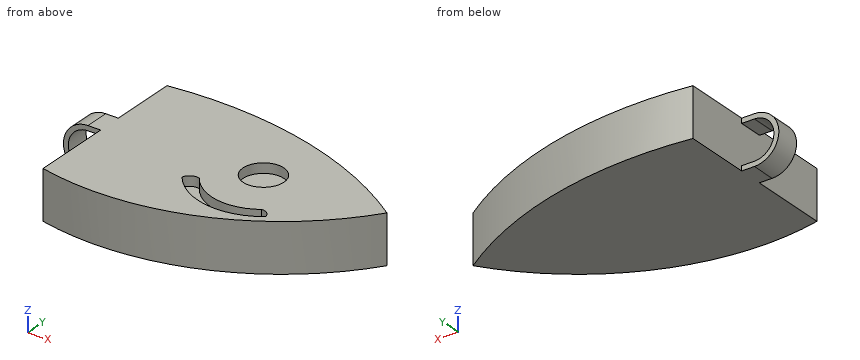
```python
from build123d import *

# Parameters (mm, degrees)
EXTRUDE_1_DEPTH     = 10
SKETCH_2_R          = 4.182683646
CUT_EXTRUDE_1_DEPTH = 2
CUT_EXTRUDE_2_DEPTH = 2
EXTRUDE_2_DEPTH     = 5
CUT_EXTRUDE_4_DEPTH = 5


with BuildPart() as part:
    # 草圖1 → 填料-伸長1 (new body)
    with BuildSketch(Plane.XY):
        with BuildLine():
            Line((-54.969523774, 13.719179235), (-54.969523774, -21.22476033))
            ThreePointArc((-54.969523774, -21.22476033), (-24.214711694, -19.081408744), (0, 0))
            ThreePointArc((0, 0), (-26.203666434, 11.992637721), (-54.969523774, 13.719179235))
        make_face()
    extrude(amount=EXTRUDE_1_DEPTH)

    # 草圖2 → 除料-伸長1 (cut)
    with BuildSketch(Plane(origin=(-3.59892411, 0, 10), x_dir=(1, 0, 0), z_dir=(0, 0, 1))):
        with Locations((-20.534055943, -1.585781503)):
            Circle(SKETCH_2_R)
    extrude(amount=-CUT_EXTRUDE_1_DEPTH, mode=Mode.SUBTRACT)

    # 草圖3 → 除料-伸長2 (cut)
    with BuildSketch(Plane(origin=(-4.498655138, 1.869163063, 10), x_dir=(1, 0, 0), z_dir=(0, 0, 1))):
        with BuildLine():
            ThreePointArc((-30.154301824, -11.927771695), (-21.15958892, -17.29086396), (-11.007087523, -14.722920379))
            ThreePointArc((-11.007087523, -14.722920379), (-11.654774806, -13.513501992), (-12.967946819, -13.116298119))
            ThreePointArc((-12.967946819, -13.116298119), (-20.827814666, -14.857391145), (-27.616719206, -10.530763976))
            ThreePointArc((-27.616719206, -10.530763976), (-29.174840287, -10.703717268), (-30.154301824, -11.927771695))
        make_face()
    extrude(amount=-CUT_EXTRUDE_2_DEPTH, mode=Mode.SUBTRACT)

    # 草圖4 → 填料-伸長2 (add)
    with BuildSketch(Plane(origin=(0, 0, 0), x_dir=(1, 0, 0), z_dir=(0, 1, 0))):
        with BuildLine():
            Line((-54.969523774, 0), (-57.578183819, 0))
            ThreePointArc((-57.578183819, 0), (-62.578183819, -5), (-57.578183819, -10))
            Line((-57.578183819, -10), (-54.969523774, -10))
            Line((-54.969523774, -10), (-54.969523774, 0))
        make_face()
    extrude(amount=-EXTRUDE_2_DEPTH)

    # 草圖5 → 除料-伸長4 (cut)
    with BuildSketch(Plane(origin=(0, 0, 0), x_dir=(1, 0, 0), z_dir=(0, 1, 0))):
        with BuildLine():
            Line((-54.969523774, -1), (-57.578183819, -1))
            ThreePointArc((-57.578183819, -1), (-61.578183819, -5), (-57.578183819, -9))
            Line((-57.578183819, -9), (-54.969523774, -9))
            Line((-54.969523774, -9), (-54.969523774, -1))
        make_face()
    extrude(amount=-CUT_EXTRUDE_4_DEPTH, mode=Mode.SUBTRACT)


solid = part.part
```
Model file for the job. Use its own axes, mm. Coordinates: 2 decimals unless noted, no trailing zeros. Order: outer loops, then holes, each group sorted by start corner. A loop starts at its lowest first (then second) coordinate and runs counter-clockwise, first axis right, second up. Notation, with made-up numbers: (0.25, 53.5) -> (17.25, 53.5) arc R11 cw to (17.25, 59.5) -> close; hole circle Ø3 at (17.25, 31). An arc over 180 degrees is marked (long way). Answer as a JSON object with one key per item and string values. Group by question number.
1) Cut at A-A, the plane z = 5. Write the cut outline in (x, y), then the cut area to 3 significant figures.
2) Cut at B-B, the plane x = -23.5. Write the cut outline in (y, z).
3) Cut at D-D, the plane x = -51. Write the cut outline in (y, z), then the cut area to 3 significant figures.
4) Drill centre lines: L1, parallel to Z at x = -20.5, y = -1.5; L2, parallel to Y at x = -32.5, z = 8.25; L3, parallel to X at y = -12, z = 3.75. Where is each one in solid material? Low to high.
5) Flat gauge pins, fed straight in: pin 1 (2 mm diameter, centred on x = -54, z = 3, fed in from +Y); pin 2 (1.5 mm diameter, centred on y = -7, z = 6.5, fed in from +X); pin 3 (6.5 mm diameter, centred on x = -22.5, y = -3.5, fed in from +Z); pin 4 (1.5 mm diameter, centred on y = -11, z = 2.5, fed in from -X). Where does each tip first touch, or does it go through?
6) Cut at C-C, the plane y = 9.5. Write the cut outline in (x, z), then the cut area to 3 significant figures.
Check values:
{
 "1": {"outline": "(-62.58, -5) -> (-61.58, -5) -> (-61.58, 0) -> (-62.58, 0) -> close; (-54.97, -21.22) arc R52.35 ccw to (0, 0) arc R78.49 ccw to (-54.97, 13.72) -> close", "area": "1,530 mm²"},
 "2": {"outline": "(-18.8, 0) -> (11.27, 0) -> (11.27, 10) -> (2.55, 10) -> (2.55, 8) -> (-5.72, 8) -> (-5.72, 10) -> (-13.15, 10) -> (-13.15, 8) -> (-15.56, 8) -> (-15.56, 10) -> (-18.8, 10) -> close"},
 "3": {"outline": "(-21.99, 0) -> (14.11, 0) -> (14.11, 10) -> (-21.99, 10) -> close", "area": "361 mm²"},
 "4": {"L1": "z = 0 to 8", "L2": "y = -21.52 to -12.34, -8.59 to 13.29", "L3": "x = -54.97 to -11.49"},
 "5": {"pin 1": "stops at y = 13.94", "pin 2": "stops at x = -5.07", "pin 3": "stops at z = 10", "pin 4": "stops at x = -54.97"},
 "6": {"outline": "(-54.97, 0) -> (-18.11, 0) -> (-18.11, 10) -> (-54.97, 10) -> close", "area": "369 mm²"}
}
